Verification items for the finished model (mm, model axes). A direction names the side the tool comes from. Give positions to 0.01 mm unless a question says otherwise; leave off trailing zeros. Order: outer loops, then holes, each group sorted by start corner. A loop starts at its lowest first (then second) coordinate and runs counter-clockwise, first axis right, second up.
(1) Sectioned sample at B-B on x = 6. Record the cut outline in (y, z).
(2) Sectioned sample at C-C on y = -1. Record the cut outline in (x, z).
(3) Scan lines: L1, parallel to X at y = -6.5, z = 2.95; L2, parallel to X at y = 2, z = 2.1; L3, parallel to Y at x = -1.5, z = 2.95. Record each from-to range of solid material in increasing order.
(4) Mould release check, pull along Y, two halves, no side actions. Record for faces 1 (the face through (7.929, -9.117, 2.486)), 2 (the face through (6.436, 9.825, 2.514)), 3 (the face through (0, -12.25, 2)), 4 (the face through (0, 0, 0)): pulls with the +Y half, pulls with the -Y half, needs draft (parallel to the pull), parting line crosses it, or undercut.
(5) Gauge pin test, flat ends, axial feed: pin 1 (1.5 mm diameter, centred on x = -14.5, y = 5.5, fed in from +Z); pin 2 (1 mm diameter, centred on x = 0.5, z = 2.5, fed in from -Y); pin 3 (1 mm diameter, centred on x = 4.5, z = 1.5, fed in from +Y). Record the tip position at first contact, or that the pin passes through.
(6) Sectioned sample at A-A on z = 0.75. Record the cut outline in (x, y).
(7) Access from +Z, -Z, +X, -X, +Y, -Y to the whole of each face (thin tool, end or side, straight path). Record for faces 5 (the face through (12.27, -9.29, 2.49)), 6 (the face through (-11.145, 4.623, 2.514)), 7 (the face through (13.9, 2.51, 2.49)), 8 (the face through (11.837, -3.488, 2.486)).
```python
from build123d import *
from build123d import SkipClean  # not in build123d's __all__

# Parameters (mm, degrees)
F1_DEPTH    = 1.5
F2_DEPTH    = 3.5
F3_R        = 1
F4_R        = 1
F5_T1_DEPTH = 9.63963589
F5_T3_DEPTH = 10.6906794787
F5_T5_DEPTH = 9.0103178495
F5_T7_DEPTH = 9.246443515
F5_T9_DEPTH = 9.9071921997
F6_T1_DEPTH = 4.304276514
F6_T3_DEPTH = 5.0643678136
F6_T5_DEPTH = 5.03100669
F6_T7_DEPTH = 4.8959965939


# Not quite as in the source:
# - a fillet or chamfer that OpenCascade refuses, or shapes differently, is made with other operations: its cross-section is extruded or revolved along the edge and cut away or added
# - a feature names something its author has since deleted; it is built from what else it names


with BuildPart() as f1:
    # F0 (on Top) → F1 (new body)
    with BuildSketch(Plane.XY):
        with BuildLine():
            Line((0, -12.25), (0, -16.25))
            ThreePointArc((0, -16.25), (2.3542947693, -16.0785508097), (4.6589105316, -15.5678210633))
            Line((4.6589105316, -15.5678210633), (3, -12.25))
            Line((3, -12.25), (0, -12.25))
        make_face()
        with BuildLine():
            Line((3, -12.25), (4.6589105316, -15.5678210633))
            ThreePointArc((4.6589105316, -15.5678210633), (6.5703749152, -14.8624585272), (8.3785487777, -13.9234485807))
            Line((8.3785487777, -13.9234485807), (6.722135955, -10.0139320225))
            Line((6.722135955, -10.0139320225), (9.1300793123, -8.2245721403))
            Line((9.1300793123, -8.2245721403), (12.269716972, -10.6544143635))
            ThreePointArc((12.269716972, -10.6544143635), (13.901957351, -8.4141596021), (15.1297175637, -5.9290932226))
            Line((15.1297175637, -5.9290932226), (11.5782397372, -5.0612652418))
            Line((11.5782397372, -5.0612652418), (12.0646680977, -2.1009633231))
            Line((12.0646680977, -2.1009633231), (16.187616292, -1.4225254948))
            ThreePointArc((16.187616292, -1.4225254948), (16.2256082415, 0.890020895), (15.9349057476, 3.184537457))
            Line((15.9349057476, 3.184537457), (12.0646680977, 1.8990366769))
            Line((12.0646680977, 1.8990366769), (10.9139659303, 4.6695753469))
            Line((10.9139659303, 4.6695753469), (14.3535137791, 7.6183424833))
            ThreePointArc((14.3535137791, 7.6183424833), (13.1072409386, 9.6053492897), (11.5878961133, 11.3922413803))
            Line((11.5878961133, 11.3922413803), (8.5738108299, 7.9135966332))
            Line((8.5738108299, 7.9135966332), (6.2013811224, 9.7497821584))
            Line((6.2013811224, 9.7497821584), (7.9085498801, 14.1956802864))
            ThreePointArc((7.9085498801, 14.1956802864), (4.08550458, 15.7280371416), (0, 16.25))
            Line((0, 16.25), (0, -12.25))
            Line((0, -12.25), (3, -12.25))
        make_face()
        with BuildLine():
            Line((6.722135955, -10.0139320225), (8.3785487777, -13.9234485807))
            ThreePointArc((8.3785487777, -13.9234485807), (10.4527204974, -12.4419907653), (12.269716972, -10.6544143635))
            Line((12.269716972, -10.6544143635), (9.1300793123, -8.2245721403))
            Line((9.1300793123, -8.2245721403), (6.722135955, -10.0139320225))
        make_face()
        with BuildLine():
            ThreePointArc((11.5878961133, 11.3922413803), (9.8484856206, 12.9255495427), (7.9085498801, 14.1956802864))
            Line((7.9085498801, 14.1956802864), (6.2013811224, 9.7497821584))
            Line((6.2013811224, 9.7497821584), (8.5738108299, 7.9135966332))
            Line((8.5738108299, 7.9135966332), (11.5878961133, 11.3922413803))
        make_face()
        with BuildLine():
            Line((11.5782397372, -5.0612652418), (15.1297175637, -5.9290932226))
            ThreePointArc((15.1297175637, -5.9290932226), (15.8199601178, -3.7136722892), (16.187616292, -1.4225254948))
            Line((16.187616292, -1.4225254948), (12.0646680977, -2.1009633231))
            Line((12.0646680977, -2.1009633231), (11.5782397372, -5.0612652418))
        make_face()
        with BuildLine():
            ThreePointArc((15.9349057476, 3.184537457), (15.3056115889, 5.4590066762), (14.3535137791, 7.6183424833))
            Line((14.3535137791, 7.6183424833), (10.9139659303, 4.6695753469))
            Line((10.9139659303, 4.6695753469), (12.0646680977, 1.8990366769))
            Line((12.0646680977, 1.8990366769), (15.9349057476, 3.184537457))
        make_face()
    extrude(amount=F1_DEPTH)

    # F0 (on Top) → F2 (join)
    with BuildSketch(Plane.XY):
        with BuildLine():
            Line((3, -12.25), (4.6589105316, -15.5678210633))
            ThreePointArc((4.6589105316, -15.5678210633), (6.5703749152, -14.8624585272), (8.3785487777, -13.9234485807))
            Line((8.3785487777, -13.9234485807), (6.722135955, -10.0139320225))
            Line((6.722135955, -10.0139320225), (9.1300793123, -8.2245721403))
            Line((9.1300793123, -8.2245721403), (12.269716972, -10.6544143635))
            ThreePointArc((12.269716972, -10.6544143635), (13.901957351, -8.4141596021), (15.1297175637, -5.9290932226))
            Line((15.1297175637, -5.9290932226), (11.5782397372, -5.0612652418))
            Line((11.5782397372, -5.0612652418), (12.0646680977, -2.1009633231))
            Line((12.0646680977, -2.1009633231), (16.187616292, -1.4225254948))
            ThreePointArc((16.187616292, -1.4225254948), (16.2256082415, 0.890020895), (15.9349057476, 3.184537457))
            Line((15.9349057476, 3.184537457), (12.0646680977, 1.8990366769))
            Line((12.0646680977, 1.8990366769), (10.9139659303, 4.6695753469))
            Line((10.9139659303, 4.6695753469), (14.3535137791, 7.6183424833))
            ThreePointArc((14.3535137791, 7.6183424833), (13.1072409386, 9.6053492897), (11.5878961133, 11.3922413803))
            Line((11.5878961133, 11.3922413803), (8.5738108299, 7.9135966332))
            Line((8.5738108299, 7.9135966332), (6.2013811224, 9.7497821584))
            Line((6.2013811224, 9.7497821584), (7.9085498801, 14.1956802864))
            ThreePointArc((7.9085498801, 14.1956802864), (4.08550458, 15.7280371416), (0, 16.25))
            Line((0, 16.25), (0, -12.25))
            Line((0, -12.25), (3, -12.25))
        make_face()
    extrude(amount=F2_DEPTH)

    # F3
    f3_edges = [f1.edges().sort_by_distance(p)[0] for p in [
        (3, -12.25, 2.5),
        (9.130079, -8.224572, 2.5),
        (12.064668, -2.100963, 2.5),
        (10.913966, 4.669575, 2.5),
        (6.201381, 9.749782, 2.5),
    ]]
    fillet(f3_edges, radius=F3_R)

    # F4
    f4_edges = [f1.edges().sort_by_distance(p)[0] for p in [
        (12.064668, 1.899037, 2.5),
        (11.57824, -5.061265, 2.5),
        (6.722136, -10.013932, 2.5),
        (8.573811, 7.913597, 2.5),
    ]]
    fillet(f4_edges, radius=F4_R)

    # F5: fillet of radius 3 on 5 edges, made by hand

    # F5_s2 → F5_t1 (cut)
    with BuildSketch(Plane.XY.offset(1.5)):
        with BuildLine():
            ThreePointArc((7.4911310936, -14.4203139681), (5.1815062569, -14.6114030066), (3.4248714726, -13.0997429451))
            Line((3.4248714726, -13.0997429451), (4.6589105316, -15.5678210633))
            ThreePointArc((4.6589105316, -15.5678210633), (6.1020546546, -15.0607911144), (7.4911310936, -14.4203139681))
        make_face()
    extrude(amount=F5_T1_DEPTH, mode=Mode.SUBTRACT)

    # F5_s4 → F5_t3 (cut)
    with BuildSketch(Plane.XY.offset(1.5)):
        with BuildLine():
            ThreePointArc((14.2551270077, -7.800888026), (12.2362296702, -9.2974660849), (9.7872909338, -8.7332042566))
            Line((9.7872909338, -8.7332042566), (12.269716972, -10.6544143635))
            ThreePointArc((12.269716972, -10.6544143635), (13.3389463668, -9.2808948827), (14.2551270077, -7.800888026))
        make_face()
    extrude(amount=F5_T3_DEPTH, mode=Mode.SUBTRACT)

    # F5_s6 → F5_t5 (cut)
    with BuildSketch(Plane.XY.offset(1.5)):
        with BuildLine():
            ThreePointArc((16.1911606466, 1.381599405), (15.5696234502, -0.7158737175), (13.6891275029, -1.833655887))
            Line((13.6891275029, -1.833655887), (16.187616292, -1.4225254948))
            ThreePointArc((16.187616292, -1.4225254948), (16.2499870192, -0.0205396402), (16.1911606466, 1.381599405))
        make_face()
    extrude(amount=F5_T5_DEPTH, mode=Mode.SUBTRACT)

    # F5_s8 → F5_t7 (cut)
    with BuildSketch(Plane.XY.offset(1.5)):
        with BuildLine():
            ThreePointArc((12.7716701145, 10.0472355644), (13.3995013522, 7.899570062), (12.3664200817, 5.91478235))
            Line((12.3664200817, 5.91478235), (14.3535137791, 7.6183424833))
            ThreePointArc((14.3535137791, 7.6183424833), (13.6168564917, 8.8681294129), (12.7716701145, 10.0472355644))
        make_face()
    extrude(amount=F5_T7_DEPTH, mode=Mode.SUBTRACT)

    # F5_s10 → F5_t9 (cut)
    with BuildSketch(Plane.XY.offset(1.5)):
        with BuildLine():
            ThreePointArc((6.8847518154, 11.529451843), (6.7914209513, 13.8973561582), (5.0088339231, 15.4587865866))
            ThreePointArc((5.0088339231, 15.4587865866), (6.4894961639, 14.8979508503), (7.9085498801, 14.1956802864))
            Line((7.9085498801, 14.1956802864), (6.8847518154, 11.529451843))
        make_face()
    extrude(amount=F5_T9_DEPTH, mode=Mode.SUBTRACT)

    # F6: fillet of radius 1 on 4 edges, made by hand

    # F6_s2 → F6_t1 (cut)
    with BuildSketch(Plane.XY.offset(1.5)):
        with BuildLine():
            ThreePointArc((7.5756414815, -14.3760966936), (8.0513569254, -13.827282659), (8.0302135849, -13.1012971306))
            Line((8.0302135849, -13.1012971306), (8.3785487777, -13.9234485807))
            ThreePointArc((8.3785487777, -13.9234485807), (7.9803050872, -14.1554664605), (7.5756414815, -14.3760966936))
        make_face()
    extrude(amount=F6_T1_DEPTH, mode=Mode.SUBTRACT)

    # F6_s4 → F6_t3 (cut)
    with BuildSketch(Plane.XY.offset(1.5)):
        with BuildLine():
            ThreePointArc((14.6397584076, -7.0526572132), (14.6431333932, -6.1917144023), (13.9762230064, -5.6472289111))
            Line((13.9762230064, -5.6472289111), (15.1297175637, -5.9290932226))
            ThreePointArc((15.1297175637, -5.9290932226), (14.8953356428, -6.4954966006), (14.6397584076, -7.0526572132))
        make_face()
    extrude(amount=F6_T3_DEPTH, mode=Mode.SUBTRACT)

    # F6_s6 → F6_t5 (cut)
    with BuildSketch(Plane.XY.offset(1.5)):
        with BuildLine():
            ThreePointArc((16.1279854606, 1.9876078546), (15.6698492509, 2.7105535541), (14.82027687, 2.8143130881))
            Line((14.82027687, 2.8143130881), (15.9349057476, 3.184537457))
            ThreePointArc((15.9349057476, 3.184537457), (16.0426122647, 2.5878739778), (16.1279854606, 1.9876078546))
        make_face()
    extrude(amount=F6_T5_DEPTH, mode=Mode.SUBTRACT)

    # F6_s8 → F6_t7 (cut)
    with BuildSketch(Plane.XY.offset(1.5)):
        with BuildLine():
            ThreePointArc((10.8530428687, 10.544125571), (11.613004552, 10.8892780785), (12.3700450766, 10.5377646967))
            ThreePointArc((12.3700450766, 10.5377646967), (11.9865870504, 10.9719747942), (11.5878961133, 11.3922413803))
            Line((11.5878961133, 11.3922413803), (10.8530428687, 10.544125571))
        make_face()
    extrude(amount=F6_T7_DEPTH, mode=Mode.SUBTRACT)

    # F7: F1 across face


with BuildPart() as f1_1:
    add(f1.part, clean=False)
    with SkipClean():  # cleaning this boolean's faces spoils the solid; the shape is the same uncleaned
        add(f1.part.mirror(Plane(origin=(0, 1.0780141844, 1.6932624113), x_dir=(0, -1, 0), z_dir=(-1, 0, 0))), clean=False)


solid = f1_1.part
```
Ans:
1. outline: (-15.1, 0) - (15.1, 0) - (15.1, 1.5) - (14.91, 1.5) - (14.91, 3.5) - (-14.76, 3.5) - (-14.76, 1.5) - (-15.1, 1.5) - close
2. outline: (-16.22, 0) - (16.22, 0) - (16.22, 1.5) - (15.32, 1.5) - (15.32, 3.5) - (-15.32, 3.5) - (-15.32, 1.5) - (-16.22, 1.5) - close
3. L1: x = -14.73 to 14.73
3. L2: x = -16.13 to 16.13
3. L3: y = -12.25 to 16.18
4. face 1: undercut
4. face 2: undercut
4. face 3: pulls with the -Y half
4. face 4: needs draft
5. pin 1: stops at z = 1.5
5. pin 2: stops at y = -12.25
5. pin 3: stops at y = 15.75
6. outline: circle Ø32.5 at (0, 0)
7. face 5: +Z, -Y
7. face 6: +Z, -X
7. face 7: +Z
7. face 8: +Z, +X
